CAD build for the part. Positions are in the model's coordinates, mm. Round coordinates to 2 decimals unless told otherwise and drop trailing zeros. Order: outer loops, then holes, each group sorted by start corner. A loop starts at its lowest first (then second) coordinate and runs counter-clockwise, first axis right, second up. Notation, with made-up numbers: M -30,-3 L 7,-3 A17 ccw 7,22 Z; hole C 21,7 d7. An arc over 180 degrees is marked long. Put each result on its own line as item: value.
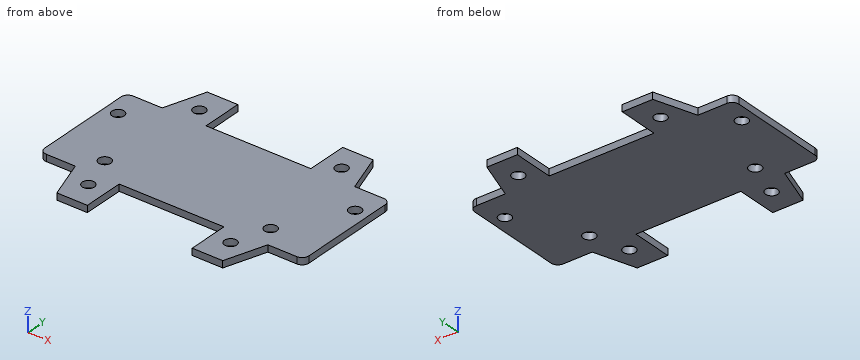
```python
from build123d import *

# Parameters (mm, degrees)
SKETCH_1_R      = 1.8
EXTRUDE_1_DEPTH = 2
FILLET_1_R      = 2


with BuildPart() as part:
    # 草图1 → 凸台-拉伸1 (new body)
    with BuildSketch(Plane.XY):
        Polygon((15.478457886, -16.428571429), (-15.478457886, -16.428571429), (-15.478457886, -28.449015282), (-24.5, -28.449015282), (-28.430563732, -16.428571429), (-39, -16.428571429), (-39, 16.428571429), (-28.430563732, 16.428571429), (-24.5, 28.449015282), (-15.478457886, 28.449015282), (-15.478457886, 16.428571429), (15.478457886, 16.428571429), (15.478457886, 28.449015282), (24.5, 28.449015282), (28.430563732, 16.428571429), (39, 16.428571429), (39, -16.428571429), (28.430563732, -16.428571429), (24.5, -28.449015282), (15.478457886, -28.449015282), align=None)
        with Locations((-21, 21)):
            Circle(SKETCH_1_R, mode=Mode.SUBTRACT)
        with Locations((21, 21)):
            Circle(SKETCH_1_R, mode=Mode.SUBTRACT)
        with Locations((24.5, -10.320512821)):
            Circle(SKETCH_1_R, mode=Mode.SUBTRACT)
        with Locations((-24.5, -10.320512821)):
            Circle(SKETCH_1_R, mode=Mode.SUBTRACT)
        with Locations((35, 8.179487179)):
            Circle(SKETCH_1_R, mode=Mode.SUBTRACT)
        with Locations((-35, 8.179487179)):
            Circle(SKETCH_1_R, mode=Mode.SUBTRACT)
        with Locations((-21, -21)):
            Circle(SKETCH_1_R, mode=Mode.SUBTRACT)
        with Locations((21, -21)):
            Circle(SKETCH_1_R, mode=Mode.SUBTRACT)
    extrude(amount=EXTRUDE_1_DEPTH)

    # 圆角1
    fillet_1_edges = [part.edges().sort_by_distance(p)[0] for p in [
        (-39, -16.428571429, 1),
        (-39, 16.428571429, 1),
        (39, 16.428571429, 1),
        (39, -16.428571429, 1),
    ]]
    fillet(fillet_1_edges, radius=FILLET_1_R)


solid = part.part
```
Item 1: Band-saw the part on B-B on x = -35. Give the cut face in (y, z).
Answers below:
outline: M -16.43,0 L 6.38,0 L 6.38,2 L -16.43,2 Z; M 9.98,0 L 16.43,0 L 16.43,2 L 9.98,2 Z
Item 2: Band-saw the part on C-C on y = 18. Give the cut face in (x, z).
Answers below:
outline: M -27.92,0 L -15.48,0 L -15.48,2 L -27.92,2 Z; M 15.48,0 L 27.92,0 L 27.92,2 L 15.48,2 Z
Item 3: Band-saw the part on A-A on x = -21. Give the cut face in (y, z), and give its area (3 significant figures).
Answers below:
outline: M -28.45,0 L -22.8,0 L -22.8,2 L -28.45,2 Z; M -19.2,0 L 19.2,0 L 19.2,2 L -19.2,2 Z; M 22.8,0 L 28.45,0 L 28.45,2 L 22.8,2 Z
area: 99.4 mm²
Item 4: Band-saw the part on D-D on z = 0.55. State how many separate pieces and enclosed holes the cut face has, and give its area (3 significant figures).
Answers below:
separate pieces: 1
enclosed holes: 8
area: 3,010 mm²
Item 5: Pin check, flat tips, straight feed: P1, Ø1, axis at x = -4, z = 1, coming from the +Y side; P2, Ø1, axis at y = 18, z = 0.5, coming from the -X side; P3, Ø2, axis at x = 35, y = 8.18, coming from the -Z side; P4, Ø0.6, axis at y = 25.5, z = 1.5, coming from the +X side. Stop position of each tip, or through.
Answers below:
P1: y = 16.43
P2: x = -28.08
P3: through
P4: x = 25.56
Item 6: Probe line 1 along X through (y, z) = (-9.5, 1.15); line 2 along Y through (x, z) = (-22, 1.4); line 3 along Y through (x, z) = (35, 0.45). List the from-to ranges inside material, lowest first. Write a range as [from, to].
Answers below:
line 1: [-39, -26.1], [-22.9, 22.9], [26.1, 39]
line 2: [-28.45, -22.5], [-19.5, 19.5], [22.5, 28.45]
line 3: [-16.43, 6.38], [9.98, 16.43]
